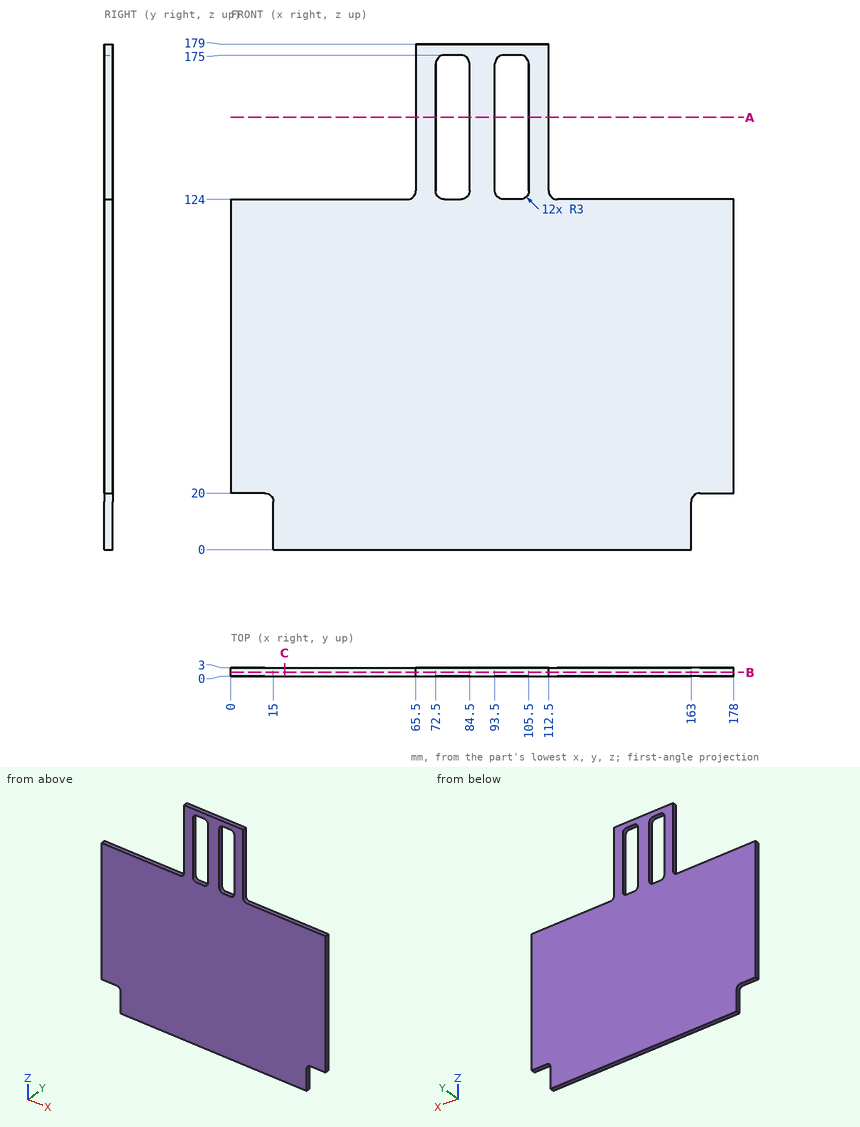
Source: three-view drawing plus pictorial views. Frame: mm from the lowest corner of the part. Give positions to 0.01 mm unless a question says otherwise; leave off trailing zeros. Write each loop counter-clockwise with the first axis right and the second up, starting at its lowest first coordinate (ties: lowest second). Pieces come first, ordered by that corner, then holes. Notation, with made-up numbers: (-39.5, -8.75) - (0.5, -8.75) arc R3 cw to (0.5, -4.75) - close; hole circle Ø10 at (-18.5, -8.5). An arc over 180 degrees is marked (long way). Write item = value, one per line. Start each with the question number.
1. Ray query, L1, parallel to X at y = 2.5, z = 156; L2, parallel to Z at x = 80, y = 2.3; L3, parallel to X at y = 1.6, z = 126. Return the intervals inside material, ascending.
2. Section query B-B, the plane y = 1.3. Count the separate pieces of the cut face and the enclosed holes in it, then the cut area to 3 significant figures.
3. Section query A-A, the plane z = 153. Output: boundary loops of the cut face in (x, y).
4. Section query C-C, the plane x = 19. Output: boundary loops of the cut face in (y, z).
5. First-contact query: pin 1 Ø1.5 at (y, z) = (1.5, 141.5) entering from +X; pin 2 Ø1.5 at (x, y) = (39.5, 1.5) entering from +Z; pin 3 Ø0.9 at (x, y) = (6, 1) entering from -Z; pin 4 Ø1 at (x, y) = (89, 1) entering from -Z. Flat tips, straight axial feed; report the tip coordinate or a pass-through.
Check sheet entries:
q1.L1 = 65.5 to 72.5, 84.5 to 93.5, 105.5 to 112.5
q1.L2 = 0 to 124, 175 to 179
q1.L3 = 65.33 to 72.67, 84.33 to 93.67, 105.33 to 112.67
q2.separate_pieces = 1
q2.enclosed_holes = 2
q2.area = 22,900 mm2
q3.outline = (65.5, 0) - (72.5, 0) - (72.5, 3) - (65.5, 3) - close; (84.5, 0) - (93.5, 0) - (93.5, 3) - (84.5, 3) - close; (105.5, 0) - (112.5, 0) - (112.5, 3) - (105.5, 3) - close
q4.outline = (0, 0) - (3, 0) - (3, 124) - (0, 124) - close
q5.pin_1 = 112.5
q5.pin_2 = 124
q5.pin_3 = 20
q5.pin_4 = 0
